Geometry check sheet. Reference: the model listing, model coordinates, mm. A direction names the side the tool comes from. Give positions to 0.01 mm unless a question says otherwise; leave off trailing zeros. Loops run counter-clockwise (first coordinate to the right, second up) from the corner with the lowest first, then second, coordinate; pieces in that order, holes last.
```python
from build123d import *


with BuildPart() as part:
    # Sketch2 → Revolve1 (revolve)
    with BuildSketch(Plane(origin=(0, 0, 0), x_dir=(0, 0, -1), z_dir=(1, 0, 0)), mode=Mode.PRIVATE) as revolve1_sk:
        with BuildLine():
            Line((0, 0), (6, 0))
            Line((6, 0), (8, 2))
            Line((8, 2), (8, 32))
            Line((8, 32), (6.5, 32))
            Line((6.5, 32), (6.5, 12.060660172))
            Line((6.5, 12.060660172), (5.378679656, 6.5))
            Line((5.378679656, 6.5), (6.5, 6.5))
            Line((6.5, 6.5), (6.5, 2.621320344))
            Line((6.5, 2.621320344), (5.378679656, 1.5))
            Line((5.378679656, 1.5), (2.65014975, 1.5))
            ThreePointArc((2.65014975, 1.5), (1.35440333, 1.91896094), (0, 2.060660172))
            Line((0, 2.060660172), (0, 0))
        make_face()
    revolve(revolve1_sk.sketch.rotate(Axis((0, 2.060660172, 0), (0, -1, 0)), 180), axis=Axis((0, 2.060660172, 0), (0, -1, 0)))


solid = part.part
```
1) Depth check by flat-ended pin: P1, Ø4, axis at y = 28, z = 2.5, coming from the -X side; P2, Ø4, axis at x = -5, y = 19, coming from the -Z side; P3, Ø6, axis at y = 3.5, z = -3.5, coming from the +X side. Enter the tip coordinate at first touch or a pass-through.
2) Tool access check on faces 1 (the flat face through (-1.3, 1.5, -2.5)), 2 (the flat face through (0, 0, 0)). Record the directions out of +Z, -Z, +X, -X, +Y, -Y that give a thin tool (end or side, any length) a straight path to the whole face; none if there is none.
3) Mould release check, pull along Z, two halves, no side actions. Record for faces 3 (the flat face through (-7, 32, 0)), 4 (the conical face through (-0.269, 0.125, -6.119)), 5 (the cylindrical face through (3.955, 4.534, -5.158)), 6 (the flat face through (-4, 6.5, 4)): +Z half, -Z half, draft (parallel to the pull), parting line (faces both ways), or undercut.
4) Sectioned sample at D-D on y = 8. Enter the section's corners in (x, z).
5) Scan lines: line 1 along X through (y, z) = (4.75, 0); line 2 along Y through (x, z) = (-1.75, -3); line 3 along X through (y, z) = (20, -4.5). Record each from-to range of solid material in increasing order.
6) Sectioned sample at A-A on x = 0. Enter the section's corners in (y, z).
7) Sectioned sample at C-C on y = 29. Enter the section's corners in (x, z).
8) Sectioned sample at B-B on z = 0. Enter the section's corners in (x, y), plus the area to 3 significant figures.
Determined:
1. P1: stops at x = -7.98
1. P2: stops at z = -7.42
1. P3: stops at x = 7.98
2. face 1: +Y
2. face 2: +Z, -Z, +X, -X, -Y
3. face 3: draft
3. face 4: parting line
3. face 5: undercut
3. face 6: undercut
4. outline: circle Ø16 at (0, 0); hole circle Ø11.36 at (0, 0)
5. line 1: x = -8 to -6.5, 6.5 to 8
5. line 2: y = 0 to 1.5
5. line 3: x = -6.61 to -4.69, 4.69 to 6.61
6. outline: (0, -6) - (2, -8) - (32, -8) - (32, -6.5) - (12.06, -6.5) - (6.5, -5.38) - (6.5, -6.5) - (2.62, -6.5) - (1.5, -5.38) - (1.5, -2.65) arc R6.54 ccw to (1.5, 2.65) - (1.5, 5.38) - (2.62, 6.5) - (6.5, 6.5) - (6.5, 5.38) - (12.06, 6.5) - (32, 6.5) - (32, 8) - (2, 8) - (0, 6) - close
7. outline: circle Ø16 at (0, 0); hole circle Ø13 at (0, 0)
8. outline: (-8, 2) - (-6, 0) - (6, 0) - (8, 2) - (8, 32) - (6.5, 32) - (6.5, 12.06) - (5.38, 6.5) - (6.5, 6.5) - (6.5, 2.62) - (5.38, 1.5) - (2.65, 1.5) arc R6.54 ccw to (-2.65, 1.5) - (-5.38, 1.5) - (-6.5, 2.62) - (-6.5, 6.5) - (-5.38, 6.5) - (-6.5, 12.06) - (-6.5, 32) - (-8, 32) - close
8. area: 121 mm2
